Autodesk Fusion 360 part; units mm, degrees
sketch "Sketch1" plane through (0, 0, 0) normal (0, 0, 1) x (1, 0, 0)
  line L0 (20.25, 10) -> (-20.25, 10)
  line L1 (-20.25, 10) -> (-20.25, -10)
  line L2 (-20.25, -10) -> (20.25, -10)
  line L3 (20.25, -10) -> (20.25, 10)
  line L4 (20.25, 10) -> (-20.25, -10) construction
  line L5 (-20.25, 10) -> (20.25, -10) construction
  dimension "d1" = 40.5
  dimension "d2" = 20
extrude "Extrude1" add sketch "Sketch1" along normal blind 8.53
sketch "Sketch2" plane through (0, 0, 8.53) normal (0, 0, 1) x (-1, 0, 0)
  line L0 (-20.25, 10) -> (-20.25, -10)
  line L1 (-20.25, -10) -> (20.25, -10)
  line L2 (20.25, -10) -> (20.25, 10)
  line L3 (20.25, 10) -> (-20.25, 10)
  line L4 (-18, -7.5) -> (18, -7.5) construction
  line L5 (18, -7.5) -> (18, 7.5) construction
  line L6 (18, 7.5) -> (-18, 7.5) construction
  line L7 (-18, 7.5) -> (-18, -7.5) construction
  line L8 (-18, -7.5) -> (18, 7.5) construction
  line L9 (18, -7.5) -> (-18, 7.5) construction
  circle A0 centre (-18, -7.5) radius 0.875
  circle A1 centre (-18, 7.5) radius 0.875
  circle A2 centre (18, 7.5) radius 0.875
  circle A3 centre (18, -7.5) radius 0.875
  dimension "d6" = 15
  dimension "d7" = 36
  dimension "d8" = 1.75
extrude "Extrude2" cut sketch "Sketch2" against normal blind 15 contours A0 | A1 | A2 | A3
sketch "Sketch3" plane through (0, 0, 8.53) normal (0, 0, 1) x (-1, 0, 0)
  circle A0 centre (-18, -7.5) radius 0.875
  circle A1 centre (-18, 7.5) radius 0.875
  circle A2 centre (18, -7.5) radius 0.875
  circle A3 centre (18, 7.5) radius 0.875
  line L0 (-20.25, 10) -> (-20.25, -10)
  line L1 (-20.25, -10) -> (20.25, -10)
  line L2 (20.25, -10) -> (20.25, 10)
  line L3 (20.25, 10) -> (-20.25, 10)
  line L4 (-18.25, -8) -> (18.25, -8)
  line L5 (18.25, -8) -> (18.25, 8)
  line L6 (18.25, 8) -> (-18.25, 8)
  line L7 (-18.25, 8) -> (-18.25, -8)
  line L8 (-18.25, -8) -> (18.25, 8) construction
  line L9 (18.25, -8) -> (-18.25, 8) construction
  circle A4 centre (-18, -7.5) radius 1.875
  circle A5 centre (-18, 7.5) radius 1.875
  circle A6 centre (18, 7.5) radius 1.875
  circle A7 centre (18, -7.5) radius 1.875
  dimension "d11" = 2
  dimension "d13" = 2
  dimension "d14" = 3.75
extrude "Extrude3" cut sketch "Sketch3" against normal blind 7.5 contours L4 L5 L6 L7 A4 A5 A6 A7
sketch "Sketch4" plane through (20.25, 0, 0) normal (1, 0, 0) x (0, 1, 0)
  line L0 (-10, 0) -> (10, 0)
  line L1 (10, 0) -> (10, 8.53)
  line L2 (10, 8.53) -> (-10, 8.53)
  line L3 (-10, 8.53) -> (-10, 0)
  line L4 (-2.5, 8.53) -> (2.5, 8.53)
  line L5 (2.5, 8.53) -> (2.5, 4.03)
  line L6 (2.5, 4.03) -> (-2.5, 4.03)
  line L7 (-2.5, 4.03) -> (-2.5, 8.53)
  dimension "d17" = 5
  dimension "d18" = 4.5
  dimension "d19" = 2.5
extrude "Extrude4" cut sketch "Sketch4" against normal blind 3 contours L2 L4 L5 L6 L7
sketch "Sketch5" plane through (0, 0, 8.53) normal (0, 0, 1) x (-1, 0, 0)
  line L0 (-20.25, 2.5) -> (-18.25, 2.5)
  line L1 (-18.25, 2.5) -> (-18.25, 5.6417)
  arc A0 (-18.25, 5.6417) -> (-16.1929, 8) centre (-18, 7.5) ccw
  line L2 (-16.1929, 8) -> (16.1929, 8)
  arc A1 (16.1929, 8) -> (18.25, 5.6417) centre (18, 7.5) ccw
  line L3 (18.25, 5.6417) -> (18.25, -5.6417)
  arc A2 (18.25, -5.6417) -> (16.1929, -8) centre (18, -7.5) ccw
  line L4 (16.1929, -8) -> (-16.1929, -8)
  arc A3 (-16.1929, -8) -> (-18.25, -5.6417) centre (-18, -7.5) ccw
  line L5 (-18.25, -5.6417) -> (-18.25, -2.5)
  line L6 (-18.25, -2.5) -> (-20.25, -2.5)
  line L7 (-20.25, -2.5) -> (-20.25, -10)
  line L8 (-20.25, -10) -> (20.25, -10)
  line L9 (20.25, -10) -> (20.25, 10)
  line L10 (20.25, 10) -> (-20.25, 10)
  line L11 (-20.25, 10) -> (-20.25, 2.5)
  circle A4 centre (-18, -7.5) radius 0.875
  circle A5 centre (-18, 7.5) radius 0.875
  circle A6 centre (18, -7.5) radius 0.875
  circle A7 centre (18, 7.5) radius 0.875
  line L12 (19.25, -9) -> (-19.25, -9)
  line L13 (-19.25, -9) -> (-19.25, 9)
  line L14 (-19.25, 9) -> (19.25, 9)
  line L15 (19.25, 9) -> (19.25, -9)
  line L16 (19.25, -9) -> (-19.25, 9) construction
  line L17 (-19.25, -9) -> (19.25, 9) construction
  dimension "d22" = 1
  dimension "d23" = 1
extrude "Extrude5" cut sketch "Sketch5" against normal blind 1 contours L0 L6 L7 L8 L9 L10 L11 L12 L13 L14 L15
fillet "Fillet1" radius 1 4 edges at (-20.25, -10, 3.765) (-20.25, 10, 3.765) (20.25, -10, 3.765) (20.25, 10, 3.765)
chamfer "Chamfer1" distance 1 angle 45 8 edges at (0, 10, 0) (-19.9571, 9.7071, 0) (-20.25, 0, 0) (-19.9571, -9.7071, 0) (0, -10, 0) (19.9571, -9.7071, 0) (20.25, 0, 0) (19.9571, 9.7071, 0)
sketch "Sketch6" plane through (0, 0, 0) normal (0, 0, -1) x (1, 0, 0)
  circle A0 centre (-18, 7.5) radius 0.875
  circle A1 centre (-18, -7.5) radius 0.875
  circle A2 centre (18, 7.5) radius 0.875
  circle A3 centre (18, -7.5) radius 0.875
  line L0 (-19.25, -9) -> (19.25, -9)
  line L1 (19.25, -9) -> (19.25, 9)
  line L2 (19.25, 9) -> (-19.25, 9)
  line L3 (-19.25, 9) -> (-19.25, -9)
  circle A4 centre (-19.25, 9) radius 5
  circle A5 centre (19.25, 9) radius 5
  circle A6 centre (19.25, -9) radius 5
  circle A7 centre (-19.25, -9) radius 5
  dimension "d29" = 10
extrude "Extrude6" cut sketch "Sketch6" against normal blind 0.5 contours L0 L3 A7 | L0 L3 A7 | L0 L1 A6 | L0 L1 A6 | L2 L3 A4 | L2 L3 A4 | L1 L2 A5 | L1 L2 A5
The listing builds one solid part. Answer for the finished solid, in the listing's coordinates (mm). A direction names the side the tool comes from. Coordinates: 2 decimals unless noted, no trailing zeros. Order: outer loops, then holes, each group sorted by start corner. A loop starts at its lowest first (then second) coordinate and runs counter-clockwise, first axis right, second up. Notation, with made-up numbers: (74.5, 87.5) -> (121.5, 87.5) arc R13 ccw to (121.5, 110.5) -> close; hole circle Ø2 at (-10, 64.25). An arc over 180 degrees is marked (long way). Answer in a Markdown table with one row per item. Add a question column.
Item 1: Each of these flat-tipped pins is pushed along its axis until it touches: P1, Ø2, axis at y = 0.5, z = 6, coming from the +X side; P2, Ø6, axis at x = 6, y = -3.5, coming from the +Z side; P3, Ø0.8, axis at y = -4, z = 8, coming from the -X side; P4, Ø1.6, axis at x = 18, y = 7.5, coming from the -Z side. Where does it stop, or does it pass through?
Item 2: Which of the six approach directions +Z, -Z, +X, -X, +Y, -Y give full straight-line access (tool end or side, diameter ignored) to faces 1 (the face through (-17, -7, 0.5)), 2 (the face through (17, 7, 0.5)), 3 (the face through (19.25, -6, 8))?
Item 3: Find section C-C (y = -7). Write down the section's boundary in (x, z).
Item 4: Find section A-A (z = 3.25). Write down the section's boundary in (x, y) (3 decimals).
Item 5: Determine the mould class of faces 4 (the face through (-20.25, 0, 4)), 5 (the face through (0, 9, 8)), 6 (the face through (0, 8, 5)) for opening direction Y: +Y half, -Y half, draft (parallel to the pull), parting line (faces both ways), or undercut.
Item 6: Find section B-B (y = -3.5). Write down the section's boundary in (x, z).
Item 7: Find the intervals of material crossed by L1, parallel to Y at x = -18, z = 5.25 (3 decimals); L2, parallel to X at y = 7.5, z = 2.5 (3 decimals); L3, parallel to Y at x = -14, z = 6, in increasing order. Write a range as from..to.
Item 8: Find section D-D (z = 5.25). Write down the section's boundary in (x, y) (3 decimals), then the cut area to 3 significant figures.
Result set:
| question | item | result |
|---|---|---|
| 1 | P1 | stops at x = -18.25 |
| 1 | P2 | stops at z = 1.03 |
| 1 | P3 | stops at x = -19.25 |
| 1 | P4 | passes through |
| 2 | face 1 | -Z, -X, -Y |
| 2 | face 2 | -Z, +X, +Y |
| 2 | face 3 | +Z, +X, +Y, -Y |
| 3 | outline | (-20.25, 1) -> (-19.75, 0.5) -> (-18.72, 0.5) -> (-18.72, 8.53) -> (-19.25, 8.53) -> (-19.25, 7.53) -> (-20.25, 7.53) -> close; (-17.28, 0.5) -> (-14.67, 0.5) -> (-14.67, 0) -> (14.67, 0) -> (14.67, 0.5) -> (17.28, 0.5) -> (17.28, 8.53) -> (16.19, 8.53) -> (16.19, 1.03) -> (-16.19, 1.03) -> (-16.19, 8.53) -> (-17.28, 8.53) -> close; (18.72, 0.5) -> (19.75, 0.5) -> (20.25, 1) -> (20.25, 7.53) -> (19.25, 7.53) -> (19.25, 8.53) -> (18.72, 8.53) -> close |
| 4 | outline | (-20.25, -9) arc R1 ccw to (-19.25, -10) -> (19.25, -10) arc R1 ccw to (20.25, -9) -> (20.25, 9) arc R1 ccw to (19.25, 10) -> (-19.25, 10) arc R1 ccw to (-20.25, 9) -> close; hole circle Ø1.75 at (-18, -7.5); hole circle Ø1.75 at (-18, 7.5); hole (-18.25, -5.642) arc R1.875 cw to (-16.193, -8) -> (16.193, -8) arc R1.875 cw to (18.25, -5.642) -> (18.25, 5.642) arc R1.875 cw to (16.193, 8) -> (-16.193, 8) arc R1.875 cw to (-18.25, 5.642) -> close; hole circle Ø1.75 at (18, -7.5); hole circle Ø1.75 at (18, 7.5) |
| 5 | face 4 | draft |
| 5 | face 5 | +Y half |
| 5 | face 6 | undercut |
| 6 | outline | (-20.25, 1) -> (-19.25, 0) -> (19.25, 0) -> (20.25, 1) -> (20.25, 7.53) -> (19.25, 7.53) -> (19.25, 8.53) -> (18.25, 8.53) -> (18.25, 1.03) -> (-18.25, 1.03) -> (-18.25, 8.53) -> (-19.25, 8.53) -> (-19.25, 7.53) -> (-20.25, 7.53) -> close |
| 7 | L1 | y = -10..-8.375, -6.625..-5.625, 5.625..6.625, 8.375..10 |
| 7 | L2 | x = -20.25..-18.875, -17.125..-16.125, 16.125..17.125, 18.875..20.25 |
| 7 | L3 | y = -10..-8, 8..10 |
| 8 | outline | (-20.25, -9) arc R1 ccw to (-19.25, -10) -> (19.25, -10) arc R1 ccw to (20.25, -9) -> (20.25, -2.5) -> (18.25, -2.5) -> (18.25, -5.642) arc R1.875 ccw to (16.193, -8) -> (-16.193, -8) arc R1.875 ccw to (-18.25, -5.642) -> (-18.25, 5.642) arc R1.875 ccw to (-16.193, 8) -> (16.193, 8) arc R1.875 ccw to (18.25, 5.642) -> (18.25, 2.5) -> (20.25, 2.5) -> (20.25, 9) arc R1 ccw to (19.25, 10) -> (-19.25, 10) arc R1 ccw to (-20.25, 9) -> close; hole circle Ø1.75 at (-18, -7.5); hole circle Ø1.75 at (-18, 7.5); hole circle Ø1.75 at (18, -7.5); hole circle Ø1.75 at (18, 7.5) |
| 8 | area | 223 mm² |
